from build123d import *

# Parameters (mm, degrees)
SCHIZZO1_R                   = 23.85
ESTRUSIONE_ESTRUSIONE1_DEPTH = 0.8
SCHIZZO2_R                   = 22.475
ESTRUSIONE_ESTRUSIONE2_DEPTH = 5.5
SCHIZZO3_R                   = 23.85
ESTRUSIONE_ESTRUSIONE3_DEPTH = 1.02
SCHIZZO4_R                   = 20.665
TAGLIO_ESTRUSIONE1_DEPTH     = 1.27
SCHIZZO5_R                   = 16.975
TAGLIO_ESTRUSIONE2_DEPTH     = 0.97
SCHIZZO6_R                   = 7.95
TAGLIO_ESTRUSIONE3_DEPTH     = 35.109403396
SCHIZZO7_R                   = 14.125
TAGLIO_ESTRUSIONE4_DEPTH     = 2.8
SCHIZZO10_R                  = 1.475
TAGLIO_ESTRUSIONE5_DEPTH     = 35.109403396


with BuildPart() as part:
    # Schizzo1 → Estrusione-Estrusione1 (new body)
    with BuildSketch(Plane.XY):
        Circle(SCHIZZO1_R)
    extrude(amount=ESTRUSIONE_ESTRUSIONE1_DEPTH)

    # Schizzo2 → Estrusione-Estrusione2 (add)
    with BuildSketch(Plane.XY.offset(0.8)):
        Circle(SCHIZZO2_R)
    extrude(amount=ESTRUSIONE_ESTRUSIONE2_DEPTH)

    # Schizzo3 → Estrusione-Estrusione3 (add)
    with BuildSketch(Plane.XY.offset(6.3)):
        Circle(SCHIZZO3_R)
    extrude(amount=ESTRUSIONE_ESTRUSIONE3_DEPTH)

    # Schizzo4 → Taglio-Estrusione1 (cut)
    with BuildSketch(Plane(origin=(0, 0, 0), x_dir=(-1, 0, 0), z_dir=(0, 0, -1))):
        Circle(SCHIZZO4_R)
    extrude(amount=-TAGLIO_ESTRUSIONE1_DEPTH, mode=Mode.SUBTRACT)

    # Schizzo5 → Taglio-Estrusione2 (cut)
    with BuildSketch(Plane(origin=(0, 0, 1.27), x_dir=(-1, 0, 0), z_dir=(0, 0, -1))):
        Circle(SCHIZZO5_R)
    extrude(amount=-TAGLIO_ESTRUSIONE2_DEPTH, mode=Mode.SUBTRACT)

    # Schizzo6 → Taglio-Estrusione3 (cut, through all)
    with BuildSketch(Plane(origin=(0, 0, 2.24), x_dir=(-1, 0, 0), z_dir=(0, 0, -1))):
        Circle(SCHIZZO6_R)
    extrude(amount=-TAGLIO_ESTRUSIONE3_DEPTH, mode=Mode.SUBTRACT)

    # Schizzo7 → Taglio-Estrusione4 (cut)
    with BuildSketch(Plane.XY.offset(7.32)):
        Circle(SCHIZZO7_R)
    extrude(amount=-TAGLIO_ESTRUSIONE4_DEPTH, mode=Mode.SUBTRACT)

    # Schizzo10 → Taglio-Estrusione5 (cut, through all)
    with BuildSketch(Plane(origin=(0, 0, 2.24), x_dir=(-1, 0, 0), z_dir=(0, 0, -1))):
        with Locations((0, 10.65)):
            Circle(SCHIZZO10_R)
        with Locations((9.22317055, 5.325)):
            Circle(SCHIZZO10_R)
        with Locations((9.22317055, -5.325)):
            Circle(SCHIZZO10_R)
        with Locations((0, -10.65)):
            Circle(SCHIZZO10_R)
        with Locations((-9.22317055, -5.325)):
            Circle(SCHIZZO10_R)
        with Locations((-9.22317055, 5.325)):
            Circle(SCHIZZO10_R)
        with BuildLine():
            Line((-12.12588027, 2.5), (-12.12588027, -2.5))
            ThreePointArc((-12.12588027, -2.5), (-11.513178605, -3.421954446), (-10.42588027, -3.214142843))
            Line((-10.42588027, -3.214142843), (-9.354666006, -2.164142843))
            ThreePointArc((-9.354666006, -2.164142843), (-9.13271156, -1.837298335), (-9.054666006, -1.45))
            Line((-9.054666006, -1.45), (-9.054666006, 1.45))
            ThreePointArc((-9.054666006, 1.45), (-9.13271156, 1.837298335), (-9.354666006, 2.164142843))
            Line((-9.354666006, 2.164142843), (-10.42588027, 3.214142843))
            ThreePointArc((-10.42588027, 3.214142843), (-11.513178605, 3.421954446), (-12.12588027, 2.5))
        make_face()
        with BuildLine():
            Line((-2.429410782, 10.636148592), (-2.803130324, 9.183449827))
            ThreePointArc((-2.803130324, 9.183449827), (-2.975208748, 8.827809384), (-3.271596168, 8.566570784))
            Line((-3.271596168, 8.566570784), (-5.783069839, 7.116570784))
            ThreePointArc((-5.783069839, 7.116570784), (-6.157502812, 6.990511049), (-6.551535682, 7.019306984))
            Line((-6.551535682, 7.019306984), (-7.996469488, 7.42200575))
            ThreePointArc((-7.996469488, 7.42200575), (-8.720088783, 8.259727927), (-8.228003645, 9.251320357))
            Line((-8.228003645, 9.251320357), (-3.897876626, 11.751320357))
            ThreePointArc((-3.897876626, 11.751320357), (-2.793089822, 11.681682373), (-2.429410782, 10.636148592))
        make_face()
        with BuildLine():
            Line((7.996469488, 7.42200575), (6.551535682, 7.019306984))
            ThreePointArc((6.551535682, 7.019306984), (6.157502812, 6.990511049), (5.783069839, 7.116570784))
            Line((5.783069839, 7.116570784), (3.271596168, 8.566570784))
            ThreePointArc((3.271596168, 8.566570784), (2.975208748, 8.827809384), (2.803130324, 9.183449827))
            Line((2.803130324, 9.183449827), (2.429410782, 10.636148592))
            ThreePointArc((2.429410782, 10.636148592), (2.793089822, 11.681682373), (3.897876626, 11.751320357))
            Line((3.897876626, 11.751320357), (8.228003645, 9.251320357))
            ThreePointArc((8.228003645, 9.251320357), (8.720088783, 8.259727927), (7.996469488, 7.42200575))
        make_face()
        with BuildLine():
            Line((10.42588027, -3.214142843), (9.354666006, -2.164142843))
            ThreePointArc((9.354666006, -2.164142843), (9.13271156, -1.837298335), (9.054666006, -1.45))
            Line((9.054666006, -1.45), (9.054666006, 1.45))
            ThreePointArc((9.054666006, 1.45), (9.13271156, 1.837298335), (9.354666006, 2.164142843))
            Line((9.354666006, 2.164142843), (10.42588027, 3.214142843))
            ThreePointArc((10.42588027, 3.214142843), (11.513178605, 3.421954446), (12.12588027, 2.5))
            Line((12.12588027, 2.5), (12.12588027, -2.5))
            ThreePointArc((12.12588027, -2.5), (11.513178605, -3.421954446), (10.42588027, -3.214142843))
        make_face()
        with BuildLine():
            Line((2.429410782, -10.636148592), (2.803130324, -9.183449827))
            ThreePointArc((2.803130324, -9.183449827), (2.975208748, -8.827809384), (3.271596168, -8.566570784))
            Line((3.271596168, -8.566570784), (5.783069839, -7.116570784))
            ThreePointArc((5.783069839, -7.116570784), (6.157502812, -6.990511049), (6.551535682, -7.019306984))
            Line((6.551535682, -7.019306984), (7.996469488, -7.42200575))
            ThreePointArc((7.996469488, -7.42200575), (8.720088783, -8.259727927), (8.228003645, -9.251320357))
            Line((8.228003645, -9.251320357), (3.897876626, -11.751320357))
            ThreePointArc((3.897876626, -11.751320357), (2.793089822, -11.681682373), (2.429410782, -10.636148592))
        make_face()
        with BuildLine():
            Line((-7.996469488, -7.42200575), (-6.551535682, -7.019306984))
            ThreePointArc((-6.551535682, -7.019306984), (-6.157502812, -6.990511049), (-5.783069839, -7.116570784))
            Line((-5.783069839, -7.116570784), (-3.271596168, -8.566570784))
            ThreePointArc((-3.271596168, -8.566570784), (-2.975208748, -8.827809384), (-2.803130324, -9.183449827))
            Line((-2.803130324, -9.183449827), (-2.429410782, -10.636148592))
            ThreePointArc((-2.429410782, -10.636148592), (-2.793089822, -11.681682373), (-3.897876626, -11.751320357))
            Line((-3.897876626, -11.751320357), (-8.228003645, -9.251320357))
            ThreePointArc((-8.228003645, -9.251320357), (-8.720088783, -8.259727927), (-7.996469488, -7.42200575))
        make_face()
    extrude(amount=-TAGLIO_ESTRUSIONE5_DEPTH, mode=Mode.SUBTRACT)


solid = part.part
Verification items for the finished model (mm, model axes). A direction names the side the tool comes from. Round coordinates to 2 decimals unless told otherwise and drop trailing zeros. Loops run counter-clockwise (first coordinate to the right, second up) from the corner with the lowest first, then second, coordinate; pieces in that order, holes last. Notation, with made-up numbers: (14, 78.25) - (29, 78.25) arc R19 cw to (29, 90.25) - close; hole circle Ø9 at (-24, 53). An arc over 180 degrees is marked (long way). Use one line per item in the form item = value.
1. Access from +Z, -Z, +X, -X, +Y, -Y to the whole of each face (thin tool, end or side, straight path). Record for faces 5 (the flat face through (-3.53, -7.31, 2.24)), 6 (the flat face through (10.3, -10.3, 7.32)), 7 (the cylindrical face through (8.718, 8.243, 3.364)), 8 (the flat face through (-16, 16, 6.3)).
A:
face_5 = -Z
face_6 = +Z, +X, -X, +Y, -Y
face_7 = +Z, -Z
face_8 = none
2. Section check C-C on z = 5.5. Record the cut outline in (x, y) (3 decimals), and give its area (3 significant figures).
A:
outline = circle Ø44.95 at (0, 0); hole circle Ø28.25 at (0, 0)
area = 960 mm²
3. Gauge pin test, flat ends, axial feed: pin 1 Ø4 at (y, z) = (-2.5, 6) entering from +X; pin 2 Ø4.5 at (x, y) = (0, -10.65) entering from -Z; pin 3 Ø4 at (y, z) = (-8.5, 5) entering from -X. Record the tip position at first contact, or that the pin passes through.
A:
pin_1 = 23.84
pin_2 = 2.24
pin_3 = -22.81
4. Scan lines: probe 1 along Y at (x, z) = (0, 3.7) (3 decimals); probe 2 along Y at (x, z) = (-9, 3.25); probe 3 along Y at (x, z) = (4.5, 3.5). Record each from-to range of solid material in increasing order.
A:
probe_1 = -22.475 to -12.125, -9.175 to -7.95, 7.95 to 9.175, 12.125 to 22.475
probe_2 = -20.59 to -6.78, -3.87 to 3.87, 6.78 to 20.59
probe_3 = -22.02 to -11.4, -7.86 to -6.55, 6.55 to 7.86, 11.4 to 22.02
5. Draft check along X on faces 1 (the cylindrical face through (7.594, 11.91, 5.94)), 2 (the flat face through (-7, 20, 0)), 3 (the flat face through (3, 17, 1.27)), 4 (the cylindrical face through (22.75, 7.16, 6.8)). Enter one of: pulls with the +X half, pulls with the -X half, needs draft (parallel to the pull), parting line crosses it, or undercut.
A:
face_1 = undercut
face_2 = needs draft
face_3 = undercut
face_4 = parting line crosses it
6. Section check B-B on y = 0. Give the number of separate pieces and of enclosed holes in the cut face, and give its area (3 significant figures).
A:
separate_pieces = 4
enclosed_holes = 0
area = 119 mm²
7. Section check A-A on x = -19.5. Record the cut outline in (y, z).
A:
outline = (-13.73, 0) - (-6.84, 0) - (-6.84, 1.27) - (6.84, 1.27) - (6.84, 0) - (13.73, 0) - (13.73, 0.8) - (11.17, 0.8) - (11.17, 6.3) - (13.73, 6.3) - (13.73, 7.32) - (-13.73, 7.32) - (-13.73, 6.3) - (-11.17, 6.3) - (-11.17, 0.8) - (-13.73, 0.8) - close
